Geometry: final body of the model. Coordinates: model frame, mm. Face numbers are marked on the shaded views. A direction names the side the tool comes from. Round coordinates to 2 decimals unless told otherwise and drop trailing zeros. Loops run counter-clockwise (first coordinate to the right, second up) from the corner with the lowest first, then second, coordinate; pieces in that order, holes last. Notation, with made-up numbers: M 16.25,28 L 21.25,28 A28 cw 21.25,54 Z; hole C 27.5,84.25 d9. An arc over 180 degrees is marked long. Answer as a JSON object with one key per item and string values.
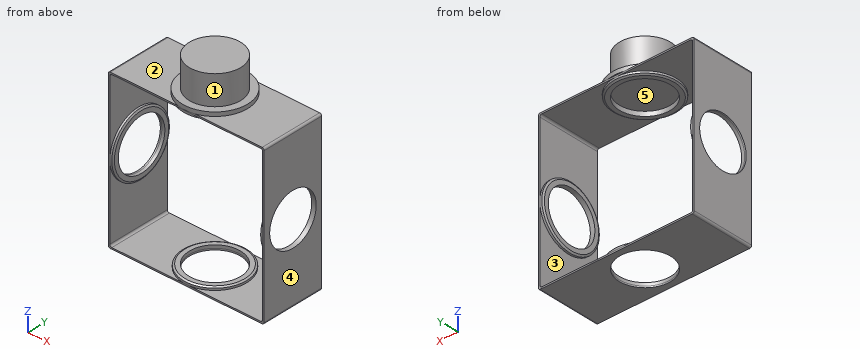
from build123d import *
from OCP.BRepFilletAPI import BRepFilletAPI_MakeChamfer

# Parameters (mm, degrees)
EXTRUDE_1_DEPTH     = 63
CUT_EXTRUDE_1_REACH = 230.077
SKETCH_2_R          = 25.5
CUT_EXTRUDE_2_REACH = 230.077
SKETCH_3_R          = 25.5
SKETCH_4_R          = 31.5
SKETCH_4_R_2        = 25.5
EXTRUDE_1_2_DEPTH   = 3
CHAMFER_1_SIZE      = 1
CHAMFER_1_SIZE2     = 1.732050808
SKETCH_5_R          = 31.5
SKETCH_5_R_2        = 25.5
EXTRUDE_4_DEPTH     = 3
CHAMFER_2_SIZE      = 1
CHAMFER_2_SIZE2     = 1.732050808
SKETCH_7_R          = 31.5
SKETCH_7_R_2        = 25.5
EXTRUDE_5_DEPTH     = 3
SKETCH_8_R          = 31.5
SKETCH_8_R_2        = 25.5
EXTRUDE_6_DEPTH     = 3
CHAMFER_3_SIZE      = 1
CHAMFER_3_SIZE2     = 1.732050808
SKETCH_9_R          = 32.5
EXTRUDE_7_DEPTH     = 4
SKETCH_10_R         = 25.5
EXTRUDE_8_DEPTH     = 29


with BuildPart() as part:
    # Эскиз1 → Extrude 1 (new body)
    with BuildSketch(Plane(origin=(0, 0, 0), x_dir=(1, 0, 0), z_dir=(0, 1, 0))):
        with BuildLine():
            Line((2, 0), (153, 0))
            ThreePointArc((153, 0), (154.414213562, 0.585786438), (155, 2))
            Line((155, 2), (155, 153))
            ThreePointArc((155, 153), (154.414213562, 154.414213562), (153, 155))
            Line((153, 155), (2, 155))
            ThreePointArc((2, 155), (0.585786438, 154.414213562), (0, 153))
            Line((0, 153), (0, 2))
            ThreePointArc((0, 2), (0.585786438, 0.585786438), (2, 0))
        make_face()
        with BuildLine():
            Line((3.5, 153.5), (151.5, 153.5))
            ThreePointArc((151.5, 153.5), (152.914213562, 152.914213562), (153.5, 151.5))
            Line((153.5, 151.5), (153.5, 3.5))
            ThreePointArc((153.5, 3.5), (152.914213562, 2.085786438), (151.5, 1.5))
            Line((151.5, 1.5), (3.5, 1.5))
            ThreePointArc((3.5, 1.5), (2.085786438, 2.085786438), (1.5, 3.5))
            Line((1.5, 3.5), (1.5, 151.5))
            ThreePointArc((1.5, 151.5), (2.085786438, 152.914213562), (3.5, 153.5))
        make_face(mode=Mode.SUBTRACT)
    extrude(amount=EXTRUDE_1_DEPTH)

    # Вырез-Вытянуть1: up to this face of the body (flat: up to its plane)
    cut_extrude_1_end = Plane(part.part.faces().sort_by_distance((77.5, 31.5, -155))[0])
    # Эскиз2 → Вырез-Вытянуть1 (cut, up to the picked face)
    with BuildSketch(Plane.XY, mode=Mode.PRIVATE) as cut_extrude_1_sk1:
        with Locations((77.5, 31.5)):
            Circle(SKETCH_2_R)
    cut_extrude_1_tool1 = split(extrude(cut_extrude_1_sk1.sketch, amount=-CUT_EXTRUDE_1_REACH, mode=Mode.PRIVATE), bisect_by=cut_extrude_1_end, keep=Keep.BOTH, mode=Mode.PRIVATE)
    add(cut_extrude_1_tool1.solids().sort_by(Axis((77.5, 31.5, 0), (0, 0, -1)))[0], mode=Mode.SUBTRACT)

    # Вырез-Вытянуть2: up to this face of the body (flat: up to its plane)
    cut_extrude_2_end = Plane(part.part.faces().sort_by_distance((0, 31.5, -77.5))[0])
    # Эскиз3 → Вырез-Вытянуть2 (cut, up to the picked face)
    with BuildSketch(Plane(origin=(155, 0, 0), x_dir=(0, 0, -1), z_dir=(1, 0, 0)), mode=Mode.PRIVATE) as cut_extrude_2_sk1:
        with Locations((77.5, 31.5)):
            Circle(SKETCH_3_R)
    cut_extrude_2_tool1 = split(extrude(cut_extrude_2_sk1.sketch, amount=-CUT_EXTRUDE_2_REACH, mode=Mode.PRIVATE), bisect_by=cut_extrude_2_end, keep=Keep.BOTH, mode=Mode.PRIVATE)
    add(cut_extrude_2_tool1.solids().sort_by(Axis((155, 31.5, -77.5), (-1, 0, 0)))[0], mode=Mode.SUBTRACT)

    # Эскиз4 → Extrude 1 2 (add)
    with BuildSketch(Plane(origin=(0, 0, -1.5), x_dir=(-1, 0, 0), z_dir=(0, 0, -1))):
        with Locations(Location((-77.5, 31.5, 0), (0, 0, 270))):
            Circle(SKETCH_4_R)
        with Locations(Location((-77.5, 31.5, 0), (0, 0, 180))):
            Circle(SKETCH_4_R_2, mode=Mode.SUBTRACT)
    extrude(amount=EXTRUDE_1_2_DEPTH)

    # Фаска1 шайба
    chamfer_1_edges = [part.edges().sort_by_distance(p)[0] for p in [
        (77.5, 63, -4.5),
    ]]
    chamfer_1_side = [part.faces().sort_by_distance(p)[0] for p in [
        (77.5, 63, -3),
    ]]
    chamfer(chamfer_1_edges, length=CHAMFER_1_SIZE, length2=CHAMFER_1_SIZE2, reference=chamfer_1_side[0])

    # Эскиз5 → Бобышка-Вытянуть4 (add)
    with BuildSketch(Plane(origin=(1.5, 0, 0), x_dir=(0, 0, -1), z_dir=(1, 0, 0))):
        with Locations(Location((77.5, 31.5, 0), (0, 0, 270))):
            Circle(SKETCH_5_R)
        with Locations((77.5, 31.5)):
            Circle(SKETCH_5_R_2, mode=Mode.SUBTRACT)
    extrude(amount=EXTRUDE_4_DEPTH)

    # Фаска2
    chamfer_2_edges = [part.edges().sort_by_distance(p)[0] for p in [
        (4.5, 63, -77.5),
    ]]
    chamfer_2_side = [part.faces().sort_by_distance(p)[0] for p in [
        (3, 63, -77.5),
    ]]
    chamfer(chamfer_2_edges, length=CHAMFER_2_SIZE, length2=CHAMFER_2_SIZE2, reference=chamfer_2_side[0])

    # Эскиз7 → Бобышка-Вытянуть5 (add)
    with BuildSketch(Plane.XY.offset(-153.5)):
        with Locations(Location((77.5, 31.5, 0), (0, 0, 270))):
            Circle(SKETCH_7_R)
        with Locations((77.5, 31.5)):
            Circle(SKETCH_7_R_2, mode=Mode.SUBTRACT)
    extrude(amount=EXTRUDE_5_DEPTH)

    # Эскиз8 → Бобышка-Вытянуть6 (add)
    with BuildSketch(Plane.ZY.offset(-153.5)):
        with Locations(Location((-77.5, 31.5, 0), (0, 0, 270))):
            Circle(SKETCH_8_R)
        with Locations(Location((-77.5, 31.5, 0), (0, 0, 180))):
            Circle(SKETCH_8_R_2, mode=Mode.SUBTRACT)
    extrude(amount=EXTRUDE_6_DEPTH)

    # Фаска3: one chamfer whose edges measure the first distance from different faces: ONE call of the kernel's chamfer builder (chamfer() names one face for all edges)
    chamfer_3_edges_1 = [part.edges().sort_by_distance(p)[0] for p in [
        (150.5, 63, -77.5),
    ]]
    chamfer_3_side_1 = [part.faces().sort_by_distance(p)[0] for p in [
        (152, 63, -77.5),
    ]]
    chamfer_3_edges_2 = [part.edges().sort_by_distance(p)[0] for p in [
        (77.5, 63, -150.5),
    ]]
    chamfer_3_side_2 = [part.faces().sort_by_distance(p)[0] for p in [
        (77.5, 63, -152),
    ]]
    chamfer_3 = BRepFilletAPI_MakeChamfer(part.part.solid().wrapped)
    for e in chamfer_3_edges_1:
        chamfer_3.Add(CHAMFER_3_SIZE, CHAMFER_3_SIZE2, e.wrapped, chamfer_3_side_1[0].wrapped)  # the first distance lies on this face
    for e in chamfer_3_edges_2:
        chamfer_3.Add(CHAMFER_3_SIZE, CHAMFER_3_SIZE2, e.wrapped, chamfer_3_side_2[0].wrapped)  # the first distance lies on this face
    add(Compound.cast(chamfer_3.Shape()), mode=Mode.REPLACE)

    # Эскиз9 → Бобышка-Вытянуть7 (add)
    with BuildSketch(Plane.XY):
        with Locations(Location((77.5, 31.5, 0), (0, 0, 104.250032698))):
            Circle(SKETCH_9_R)
    extrude(amount=EXTRUDE_7_DEPTH)

    # Эскиз10 → Бобышка-Вытянуть8 (add)
    with BuildSketch(Plane.XY.offset(4)):
        with Locations((77.5, 31.5)):
            Circle(SKETCH_10_R)
    extrude(amount=EXTRUDE_8_DEPTH)


solid = part.part
1) Pull-direction query (Z, two-part tool) for the marked faces 1, 2 and 3; classes: +Z half, -Z half, draft (parallel to the pull), parting line (faces both ways), or undercut.
Results:
{"face 1": "draft", "face 2": "+Z half", "face 3": "undercut"}
2) Section query A-A (z = -115). Return the cut outline in (x, y).
Results:
{"outline": "M 0,0 L 1.5,0 L 1.5,63 L 0,63 Z; M 153.5,0 L 155,0 L 155,63 L 153.5,63 Z"}
3) Pin query (flat end, axial travel): P1, Ø0.5, axis at x = 81, y = 63.5, coming from the -Z side; P2, Ø10, axis at x = 30, z = -7.5, coming from the +Y side; P3, Ø19, axis at y = 29, z = -24.5, coming from the -X side. Return the tip coordinate at first contact, or that it passes through.
Results:
{"P1": "z = 0", "P2": "through", "P3": "x = 0"}
4) Ray query, line 1 (Z direction, x = 151.7, y = 31.5); line 2 (X direction, y = 8.5, z = -120); line 3 (Y direction, x = 2, z = -77). Return the intervals inside material, ascending.
Results:
{"line 1": "-155 to -153.49, -109 to -103, -52 to -46, -1.51 to 0", "line 2": "0 to 1.5, 153.5 to 155", "line 3": "0 to 6, 57 to 63"}
5) Section query B-B (x = 17.5). Return the cut outline in (y, z).
Results:
{"outline": "M 0,-155 L 63,-155 L 63,-153.5 L 0,-153.5 Z; M 0,-1.5 L 63,-1.5 L 63,0 L 0,0 Z"}
6) Section query C-C (y = 31.5). Count the separate pieces of the cut face and the enclosed holes in it, and give its area (3 significant figures).
Results:
{"separate pieces": "3", "enclosed holes": "0", "area": "2,490 mm2"}
7) Reachability of the marked faces 4 and 5 from +Z, -Z, +X, -X, +Y, -Y: full face, straight path, thin tool, end or side. Return the list, or none.
Results:
{"face 4": "+Z, -Z, +X, +Y, -Y", "face 5": "-Z"}
